The figure shows three views and two pictorial views of one solid part (mm, origin at its lowest corner). Answer the questions. Round coordinates to 2 decimals unless told otherwise and drop trailing zeros. Write each loop counter-clockwise with the first axis right and the second up, starting at its lowest first coordinate (ties: lowest second). Pieces come first, ordered by that corner, then holes. Notation, with made-up numbers: (64.5, 82.5) -> (97.5, 82.5) arc R27 cw to (97.5, 114.5) -> close; hole circle Ø2 at (-10.5, -5). An arc over 180 degrees is marked (long way). One line per item, written item: value.
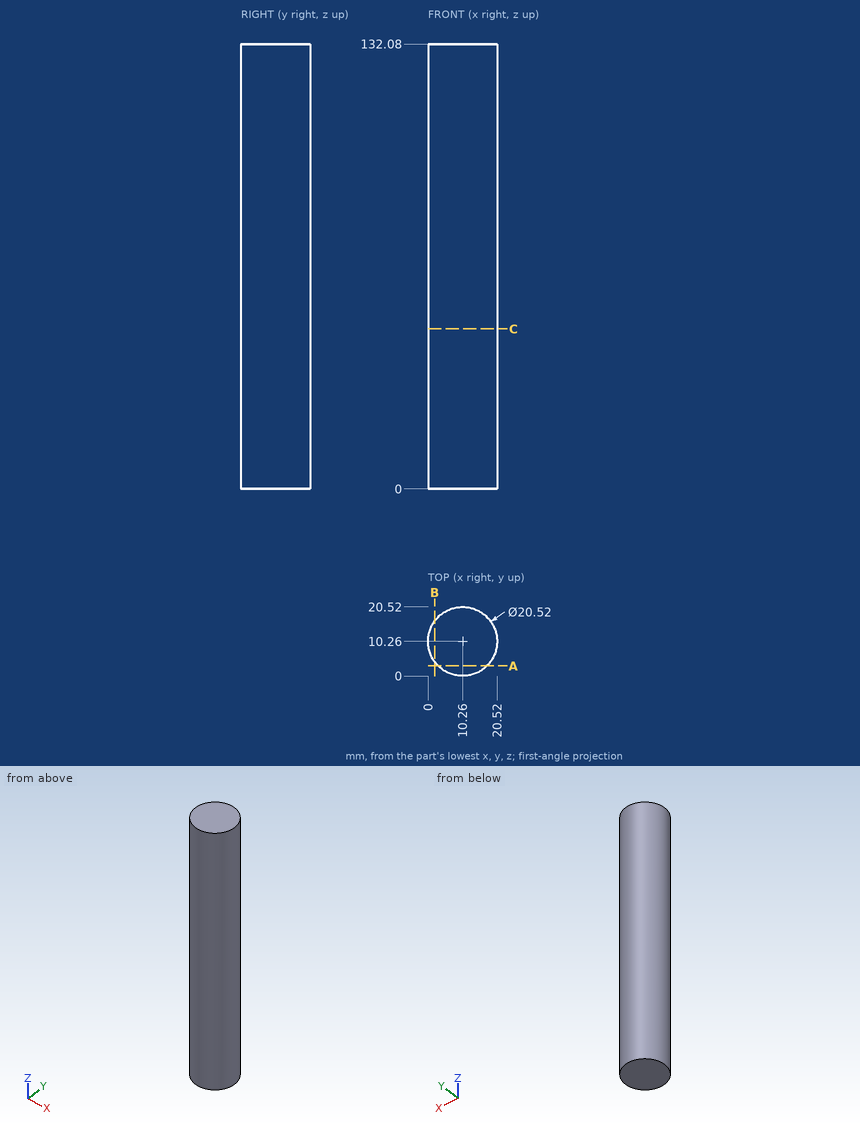
(1) Flat-ended cylindrical pins translate along their axes: pin 1 Ø4 at (y, z) = (3.5, 56.5) entering from -X; pin 2 Ø8 at (x, z) = (3.5, 18) entering from +Y; pin 3 Ø2 at (y, z) = (5.5, 61) entering from -X. Find the tip coordinate at first contact, or state that the pin passes through.
Reported:
pin 1: stops at x = 1.17
pin 2: stops at y = 20.14
pin 3: stops at x = 0.71
(2) Find section B-B on x = 2. Give the vertices of the cut face in (y, z), plus the area to 3 significant figures.
Reported:
outline: (4.17, 0) -> (16.35, 0) -> (16.35, 132.08) -> (4.17, 132.08) -> close
area: 1,610 mm2
(3) Consider probe 1 along Y at (x, z) = (16.75, 116); probe 2 along Y at (x, z) = (2.25, 126); probe 3 along X at (y, z) = (3.25, 65). Determine where each line is inside the solid, lowest interval first.
Reported:
probe 1: y = 2.31 to 18.21
probe 2: y = 3.85 to 16.67
probe 3: x = 2.77 to 17.75
(4) Find section A-A on y = 3. Give the vertices of the cut face in (x, z).
Reported:
outline: (3.01, 0) -> (17.51, 0) -> (17.51, 132.08) -> (3.01, 132.08) -> close
(5) Find section C-C on z = 47.5. Give the vertices of the cut face in (x, y).
Reported:
outline: circle Ø20.52 at (10.26, 10.26)
